```python
from build123d import *

# Parameters (mm, degrees)
ESQUISSE1_W             = 40
ESQUISSE1_H             = 8
EXTRUSION1_DEPTH        = 10
ESQUISSE2_W             = 37.4
ESQUISSE2_H             = 17.4
ENL_V_MAT_EXTRU_1_DEPTH = 5
ESQUISSE3_W             = 1.3
ESQUISSE3_H             = 4.7
ENL_V_MAT_EXTRU_2_DEPTH = 2.5
ESQUISSE4_R             = 1
ENL_V_MAT_EXTRU_3_DEPTH = 43
ENL_V_MAT_EXTRU_4_DEPTH = 1.4


with BuildPart() as part:
    # Esquisse1 → Extrusion1 (new, symmetric)
    with BuildSketch(Plane.XY):
        with Locations((20, 4)):
            Rectangle(ESQUISSE1_W, ESQUISSE1_H)
    extrude(amount=EXTRUSION1_DEPTH, both=True)

    # Esquisse2 → Enlèv. mat.-Extru.1 (cut)
    with BuildSketch(Plane(origin=(0, 8, 0), x_dir=(-1, 0, 0), z_dir=(0, 1, 0))):
        with Locations((-20, 0)):
            Rectangle(ESQUISSE2_W, ESQUISSE2_H)
    extrude(amount=-ENL_V_MAT_EXTRU_1_DEPTH, mode=Mode.SUBTRACT)

    # Esquisse3 → Enlèv. mat.-Extru.2 (cut)
    with BuildSketch(Plane(origin=(0, 8, 0), x_dir=(-1, 0, 0), z_dir=(0, 1, 0))):
        with Locations((-39.35, 0)):
            Rectangle(ESQUISSE3_W, ESQUISSE3_H)
    extrude(amount=-ENL_V_MAT_EXTRU_2_DEPTH, mode=Mode.SUBTRACT)

    # Esquisse4 → Enlèv. mat.-Extru.3 (cut, through all)
    with BuildSketch(Plane.XZ):
        with Locations(Location((37.3, 7.3, 0), (0, 0, 270))):
            Circle(ESQUISSE4_R)
        with Locations(Location((37.3, -7.3, 0), (0, 0, 270))):
            Circle(ESQUISSE4_R)
        with Locations(Location((2.7, -7.3, 0), (0, 0, 270))):
            Circle(ESQUISSE4_R)
        with Locations(Location((2.7, 7.3, 0), (0, 0, 270))):
            Circle(ESQUISSE4_R)
    extrude(amount=-ENL_V_MAT_EXTRU_3_DEPTH, mode=Mode.SUBTRACT)

    # Esquisse5 → Enlèv. mat.-Extru.4 (cut)
    with BuildSketch(Plane.XZ):
        with BuildLine():
            Line((40, -5.592893219), (36.592893219, -5.592893219))
            ThreePointArc((36.592893219, -5.592893219), (35.885786438, -5.885786438), (35.592893219, -6.592893219))
            Line((35.592893219, -6.592893219), (35.592893219, -10))
            Line((35.592893219, -10), (40, -10))
            Line((40, -10), (40, -5.592893219))
        make_face()
        with BuildLine():
            Line((40, 10), (40, 5.592893219))
            Line((40, 5.592893219), (36.592893219, 5.592893219))
            ThreePointArc((36.592893219, 5.592893219), (35.885786438, 5.885786438), (35.592893219, 6.592893219))
            Line((35.592893219, 6.592893219), (35.592893219, 10))
            Line((35.592893219, 10), (40, 10))
        make_face()
        with BuildLine():
            Line((0, 5.592893219), (3.407106781, 5.592893219))
            ThreePointArc((3.407106781, 5.592893219), (4.114213562, 5.885786438), (4.407106781, 6.592893219))
            Line((4.407106781, 6.592893219), (4.407106781, 10))
            Line((4.407106781, 10), (0, 10))
            Line((0, 10), (0, 5.592893219))
        make_face()
        with BuildLine():
            Line((0, -10), (0, -5.592893219))
            Line((0, -5.592893219), (3.407106781, -5.592893219))
            ThreePointArc((3.407106781, -5.592893219), (4.114213562, -5.885786438), (4.407106781, -6.592893219))
            Line((4.407106781, -6.592893219), (4.407106781, -10))
            Line((4.407106781, -10), (0, -10))
        make_face()
    extrude(amount=-ENL_V_MAT_EXTRU_4_DEPTH, mode=Mode.SUBTRACT)


solid = part.part
```
Verification items for the finished model (mm, model axes). A direction names the side the tool comes from. Give positions to 0.01 mm unless a question says otherwise; leave off trailing zeros. Loops run counter-clockwise (first coordinate to the right, second up) from the corner with the lowest first, then second, coordinate; pieces in that order, holes last.
1. Section check B-B, the plane y = 2. Enter the section's corners in (x, z), then the cut area to 3 significant figures.
2. Thickness scan on line 1 (X direction, y = 2.4, z = -7.3); line 2 (X direction, y = 5, z = 3.5); line 3 (Z direction, x = 7.5, y = 4.75). Record the ranges inside material, lowest first.
3. Go/stop test with flat-tipped pins: pin 1 Ø1.5 at (y, z) = (0.5, -8.5) entering from -X; pin 2 Ø1.2 at (x, z) = (2.7, 7.3) entering from -Y; pin 3 Ø3.5 at (x, z) = (38, 8) entering from -Y; pin 4 Ø1.5 at (x, z) = (16, 7.5) entering from +Y. Record where each tip stops, or that it passes through.
4. Section check D-D, the plane x = 9.5. Enter the section's corners in (y, z), then the cut area to 3 significant figures.
5. Section check A-A, the plane x = 37.3. Enter the section's corners in (y, z), then the cut area to 3 significant figures.
6. Section check C-C, the plane z = -7.3. Enter the section's corners in (x, y), then the cut area to 3 significant figures.
7. Mould release check, pull along X, two halves, no side actions. Record for faces 6 (the flat face through (4.407, 1, -8)), 7 (the flat face through (38.7, 5, 0)), 8 (the flat face through (20, 4, 10)): released by +X, released by -X, zero draft, split by the parting line, or undercut.
8. Set-up check for faces 1 (the flat face through (38.3, 1.4, -8.3)), 2 (the flat face through (1.7, 1.4, -8.3)), 3 (the flat face through (4.407, 1, 8)), 4 (the flat face through (38, 1, 5.593)), 5 (the flat face through (39, 7, 2.35)): record each of +Z, -Z, +X, -X, +Y, -Y from which the full face is reachable in a straight line by a thin tool's end or side.
Geometry says:
1. outline: (0, -10) - (40, -10) - (40, 10) - (0, 10) - close; hole circle Ø2 at (2.7, -7.3); hole circle Ø2 at (2.7, 7.3); hole circle Ø2 at (37.3, -7.3); hole circle Ø2 at (37.3, 7.3)
1. area: 787 mm2
2. line 1: x = 0 to 1.7, 3.7 to 36.3, 38.3 to 40
2. line 2: x = 0 to 1.3, 38.7 to 40
2. line 3: z = -10 to -8.7, 8.7 to 10
3. pin 1: stops at x = 4.41
3. pin 2: passes through
3. pin 3: stops at y = 1.4
3. pin 4: stops at y = 3
4. outline: (0, -10) - (8, -10) - (8, -8.7) - (3, -8.7) - (3, 8.7) - (8, 8.7) - (8, 10) - (0, 10) - close
4. area: 73.0 mm2
5. outline: (0, -5.59) - (1.4, -5.59) - (1.4, -6.3) - (3, -6.3) - (3, 6.3) - (1.4, 6.3) - (1.4, 5.59) - (0, 5.59) - close; (1.4, -10) - (8, -10) - (8, -8.7) - (3, -8.7) - (3, -8.3) - (1.4, -8.3) - close; (1.4, 8.3) - (3, 8.3) - (3, 8.7) - (8, 8.7) - (8, 10) - (1.4, 10) - close
5. area: 54.3 mm2
6. outline: (0, 1.4) - (1.7, 1.4) - (1.7, 3) - (1.3, 3) - (1.3, 8) - (0, 8) - close; (3.7, 1.4) - (4.41, 1.4) - (4.41, 0) - (35.59, 0) - (35.59, 1.4) - (36.3, 1.4) - (36.3, 3) - (3.7, 3) - close; (38.3, 1.4) - (40, 1.4) - (40, 8) - (38.7, 8) - (38.7, 3) - (38.3, 3) - close
6. area: 114 mm2
7. face 6: released by -X
7. face 7: undercut
7. face 8: zero draft
8. face 1: -Z, +X, -Y
8. face 2: -Z, -X, -Y
8. face 3: +Z, -X, -Y
8. face 4: +Z, +X, -Y
8. face 5: +X, +Y
